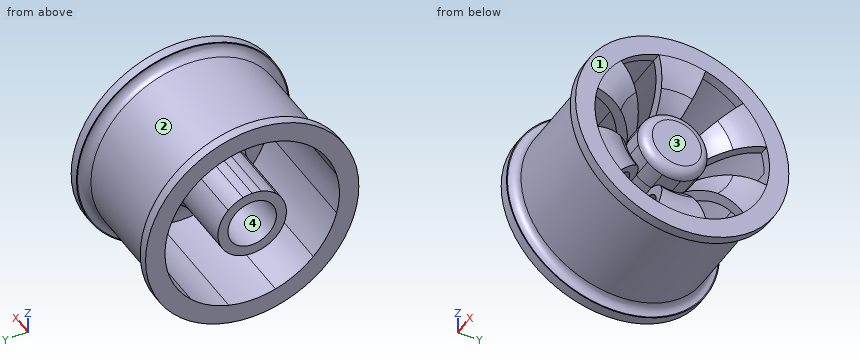
```python
from build123d import *
from build123d.topology import SkipClean

# Parameters (mm, degrees)
REVOLVE1_OUTLINE_W  = 1
REVOLVE1_OUTLINE_H  = 1
SKETCH2_R           = 3.530343639
SKETCH2_R_2         = 2.5
BOSS_EXTRUDE1_DEPTH = 13
BOSS_EXTRUDE2_START = -2
SKETCH3_R           = 3.530343639
BOSS_EXTRUDE2_DEPTH = 2
CUT_EXTRUDE1_DEPTH  = 21.928449536
CIRPATTERN1_COUNT   = 6
FILLET1_R           = 1


# Read off the part's stored shape, not the designer's step: Revolve1
with BuildPart() as part:
    # Revolve1 outline → Revolve1 (revolve)
    with BuildSketch(Plane.YX):
        with BuildLine():
            add(Edge.make_bspline(
                [(2.5, 0), (2.716234195, 0.906371087), (3.054671918, 1.91746682), (3.530343639, 2.883101851)],
                knots=[0, 0, 0, 0, 0.307599927, 0.307599927, 0.307599927, 0.307599927], degree=3))
            Line((2.5, 0), (3.530343639, 0))
            Line((3.530343639, 0), (3.530343639, 2.883101851))
        make_face()
        with BuildLine():
            add(Edge.make_bspline(
                [(3.530343639, 2.883101851), (4.125497218, 4.091290439), (4.935485854, 5.228311877), (5.989749537, 6)],
                knots=[0.307599927, 0.307599927, 0.307599927, 0.307599927, 0.692464509, 0.692464509, 0.692464509, 0.692464509], degree=3))
            Line((3.530343639, 2.883101851), (3.530343639, 0))
            add(Edge.make_bspline(
                [(9, 6), (8.813858726, 5.999997286), (8.43297149, 5.974351341), (7.749922349, 5.831183314), (6.653568172, 5.361217178), (5.311352408, 4.099132984), (4.3155593, 2.31932682), (3.78420775, 0.901212892), (3.601875729, 0.278067654), (3.530343639, 0)],
                knots=[0, 0, 0, 0, 0.0625, 0.125, 0.25, 0.5, 0.75, 0.875, 0.972909743, 0.972909743, 0.972909743, 0.972909743], degree=3))
            Line((9, 6), (5.989749537, 6))
        make_face()
        with BuildLine():
            add(Edge.make_bspline(
                [(5.989749537, 6), (6.832184813, 6.616636338), (7.830594626, 7), (9, 7)],
                knots=[0.692464509, 0.692464509, 0.692464509, 0.692464509, 1, 1, 1, 1], degree=3))
            Line((5.989749537, 6), (9, 6))
            Line((9, 6), (9, 7))
        make_face()
        Polygon((10, 6), (9, 6), (9, 0), (10, 0), (10, 5.1), align=None)
        with Locations((9.5, 6.5)):
            Rectangle(REVOLVE1_OUTLINE_W, REVOLVE1_OUTLINE_H)
        Polygon((10, 0), (9, 0), (9, -7), (10, -7), (10, -5.1), align=None)
        with BuildLine():
            Line((10.9, 6), (10, 6))
            Line((10, 6), (10, 5.1))
            ThreePointArc((10, 5.1), (10.263603897, 5.736396103), (10.9, 6))
        make_face()
        Polygon((10, 7), (10, 6), (10.9, 6), (11, 6), (11, 7), align=None)
        with BuildLine():
            Line((10, -5.1), (10, -7))
            Line((10, -7), (11, -7))
            Line((11, -7), (11, -6))
            Line((11, -6), (10.9, -6))
            ThreePointArc((10.9, -6), (10.263603897, -5.736396103), (10, -5.1))
        make_face()
    revolve(axis=Axis((0, 0, 0), (1, 0, 0)))

    # Sketch2 → Boss-Extrude1 (add)
    with BuildSketch(Plane.ZY.offset(7)):
        Circle(SKETCH2_R)
        Circle(SKETCH2_R_2, mode=Mode.SUBTRACT)
    extrude(amount=-BOSS_EXTRUDE1_DEPTH)

    # Sketch3 → Boss-Extrude2 (add)
    with BuildSketch(Plane(origin=(6, 0, 0), x_dir=(0, 0, -1), z_dir=(1, 0, 0)).offset(BOSS_EXTRUDE2_START)):
        with Locations(Location((0, 0, 0), (0, 0, 180))):
            Circle(SKETCH3_R)
    extrude(amount=BOSS_EXTRUDE2_DEPTH)

    # Sketch4 → Cut-Extrude1 (cut, through all)
    with SkipClean():  # the faces are left unmerged after this step: merging them gives an invalid solid
        with BuildSketch(Plane(origin=(7, 0, 0), x_dir=(0, 0, -1), z_dir=(1, 0, 0))):
            with BuildLine():
                Line((-0.88258591, 3.41824053), (-2.25, 8.714212529))
                ThreePointArc((-2.25, 8.714212529), (0, 9), (2.25, 8.714212529))
                Line((2.25, 8.714212529), (0.88258591, 3.41824053))
                ThreePointArc((0.88258591, 3.41824053), (0, 3.530343639), (-0.88258591, 3.41824053))
            make_face()
        cut_extrude1 = extrude(amount=-CUT_EXTRUDE1_DEPTH, mode=Mode.SUBTRACT)
    add(part.part.scale(1), mode=Mode.REPLACE)  # the faces are merged on a copy

    # CirPattern1: Cut-Extrude1 ×6 about axis
    with SkipClean():  # the faces are left unmerged after this step: merging them gives an invalid solid
        cirpattern1_axis = Axis((0, 0, 0), (1, 0, 0))
        for i in range(1, CIRPATTERN1_COUNT):
            add(cut_extrude1.rotate(cirpattern1_axis, i * 360 / CIRPATTERN1_COUNT), mode=Mode.SUBTRACT)
    add(part.part.scale(1), mode=Mode.REPLACE)  # the faces are merged on a copy

    # Fillet1
    fillet1_edges = [part.edges().sort_by_distance(p)[0] for p in [
        (6, 3.267738298, 1.336118492),
    ]]
    fillet(fillet1_edges, radius=FILLET1_R)


solid = part.part
```
CAD build for the part. Positions are in the model's coordinates, mm. Face numbers are marked on the shaded views. Round coordinates to 2 decimals unless told otherwise and drop trailing zeros. Write item = value, one per line. Start each with the question number.
Q1. Mould opens along Z. For the marked faces 1, 2, 3 and 4 say: pulls with the +Z half, pulls with the -Z half, needs draft (parallel to the pull), parting line crosses it, or undercut.
Q2. Probe L1, parallel to X at y = -9.25, z = 5.75; L2, parallel to Z at x = -0.5, y = -1.75; L3, parallel to Y at x = 1, z = 1.5. List the from-to ranges inside material, lowest first. Write a range as from..to.
Q3. Band-saw the part on A-A (z = -3). Count the separate pieces of the cut face and the enclosed holes in it, then the cut area to 3 significant figures.
Q4. Drop flat-ended pins along their axis: pin 1 (3 mm diameter, centred on x = -0.5, y = 2, fed in from +Z); pin 2 (4 mm diameter, centred on y = 1, z = 1, fed in from +X); pin 3 (3 mm diameter, centred on x = -2.5, z = -8, fed in from +Y). Give the stop position or say it passes through.
Answers below:
q1.face_1 = needs draft
q1.face_2 = parting line crosses it
q1.face_3 = undercut
q1.face_4 = undercut
q2.L1 = -7..-6, 6..7
q2.L2 = -9.85..-8.83, -3.07..-1.79, 1.79..3.07, 8.83..9.85
q2.L3 = -9.89..-8.87, -3.53..-2, 2..3.53, 8.87..9.89
q3.separate_pieces = 3
q3.enclosed_holes = 0
q3.area = 96.4 mm2
q4.pin_1 = 9.99
q4.pin_2 = 6
q4.pin_3 = 7.6
